Read the model definition and answer for the solid it produces. Units are mm, in the model's axes. A direction names the side the tool comes from. Give positions to 0.01 mm unless a question says otherwise; leave off trailing zeros. Order: outer loops, then holes, each group sorted by start corner. A loop starts at its lowest first (then second) coordinate and runs counter-clockwise, first axis right, second up.
```python
from build123d import *

# Parameters (mm, degrees)
BOSS_EXTRUDE1_DEPTH = 3.85
CHAMFER1_SIZE       = 1


with BuildPart() as part:
    # Sketch1 → Boss-Extrude1 (new body)
    with BuildSketch(Plane(origin=(0, 0, 0), x_dir=(1, 0, 0), z_dir=(0, 1, 0))):
        Polygon((20, 0), (15.9625, 6.993155136), (11.632372981, 4.493155136), (9.707372981, 7.82735294), (14.0375, 10.32735294), (10, 17.320508076), (1.925, 17.320508076), (1.925, 12.320508076), (-1.925, 12.320508076), (-1.925, 17.320508076), (-10, 17.320508076), (-14.0375, 10.32735294), (-9.707372981, 7.82735294), (-11.632372981, 4.493155136), (-15.9625, 6.993155136), (-20, 0), (-15.9625, -6.993155136), (-11.632372981, -4.493155136), (-9.707372981, -7.82735294), (-14.0375, -10.32735294), (-10, -17.320508076), (-1.925, -17.320508076), (-1.925, -12.320508076), (1.925, -12.320508076), (1.925, -17.320508076), (10, -17.320508076), (14.0375, -10.32735294), (9.707372981, -7.82735294), (11.632372981, -4.493155136), (15.9625, -6.993155136), align=None)
    extrude(amount=BOSS_EXTRUDE1_DEPTH)

    # Chamfer1
    chamfer1_edges = [part.edges().sort_by_distance(p)[0] for p in [
        (15.9625, 1.925, 6.993155136),
        (15.9625, 1.925, -6.993155136),
        (14.0375, 1.925, -10.32735294),
        (1.925, 1.925, -17.320508076),
        (-1.925, 1.925, -17.320508076),
        (-14.0375, 1.925, -10.32735294),
        (-15.9625, 1.925, -6.993155136),
        (-15.9625, 1.925, 6.993155136),
        (-14.0375, 1.925, 10.32735294),
        (-1.925, 1.925, 17.320508076),
        (1.925, 1.925, 17.320508076),
        (14.0375, 1.925, 10.32735294),
    ]]
    chamfer(chamfer1_edges, length=CHAMFER1_SIZE)


solid = part.part
```
1) For a pull along Z with two mould halves and no side action, classify faces 6 (the face through (13.39, 1.9, -5.51)), 7 (the face through (6, 2, 17.321)), 8 (the face through (-11.46, 1.9, -8.84)), 9 (the face through (0, 0, 0)) as released by +Z, released by -Z, zero draft, split by the parting line, or undercut.
Final values:
face 6: undercut
face 7: released by +Z
face 8: undercut
face 9: zero draft
2) Consider L1, parallel to Z at x = 12.5, y = 1.55; L2, parallel to X at y = 1.7, z = 6; L3, parallel to Z at x = 12, y = 1.75. Determine where each line is inside the solid, lowest interval first.
Final values:
L1: z = -12.99 to -9.44, -4.99 to 4.99, 9.44 to 12.99
L2: x = -16.54 to -14.24, -10.76 to 10.76, 14.24 to 16.54
L3: z = -13.86 to -9.15, -4.71 to 4.71, 9.15 to 13.86
3) The part is cut by section A-A on z = -14. Determine the outline of the cut face in (x, y) (3 decimals).
Final values:
outline: (-11.917, 0) - (-1.925, 0) - (-1.925, 3.85) - (-11.917, 3.85) - close; (1.925, 0) - (11.917, 0) - (11.917, 3.85) - (1.925, 3.85) - close
4) A tool of negligible diameter and unlimited length cuts with its end or side. For faces 1 (the face through (10.66, 1.9, 6.18)), 2 (the face through (13.357, 1.898, -10.52)), 3 (the face through (-13.35, 1.9, -10.5)), 4 (the face through (0, 2, -12.321)), 5 (the face through (0, 2, 12.321)), from which of +Z, -Z, +X, -X, +Y, -Y can it reach the whole face along a straight path? Write none if from no direction.
Final values:
face 1: +Y, -Y
face 2: +X, +Y, -Y
face 3: -X, +Y, -Y
face 4: -Z, +Y, -Y
face 5: +Z, +Y, -Y
5) The part is cut by section C-C on z = 3. Determine the outline of the cut face in (x, y).
Final values:
outline: (-18.27, 0) - (18.27, 0) - (18.27, 3.85) - (-18.27, 3.85) - close
6) The part is cut by section B-B on x = -0.5. Determine the outline of the cut face in (y, z).
Final values:
outline: (0, -12.32) - (3.85, -12.32) - (3.85, 12.32) - (0, 12.32) - close
7) Given pin 1 (1.2 mm diameter, centred on y = 1, z = 15, fed in from -X); pin 2 (1.9 mm diameter, centred on y = 1, z = -13.5, fed in from +X); pin 3 (1.2 mm diameter, centred on x = -0.5, y = 2.5, fed in from -Z), each flat-ended and moving along its own axis, determine where each tip first touches the part or whether it passes through.
Final values:
pin 1: stops at x = -11.69
pin 2: stops at x = 12.75
pin 3: stops at z = -12.32
